from build123d import *

# Parameters (mm, degrees)
FILLET1_R = 1.27


with BuildPart() as part:
    # Sketch1 → Revolve-Thin1 (revolve)
    with BuildSketch(Plane(origin=(0, 0, 0), x_dir=(1, 0, 0), z_dir=(0, 1, 0)), mode=Mode.PRIVATE) as revolve_thin1_sk:
        Polygon((-77.419354839, 0), (-77.419354839, 3.5), (-67.870967742, 3.5), (-67.870967742, 4), (-57.608712258, 4), (-57.608712258, 6.35), (67.904423226, 6.35), (67.904423226, 4), (76.082332903, 4), (76.082332903, 3.5), (87.741935484, 3.5), (87.741935484, 0), (85.201935484, 0), (85.201935484, 0.96), (73.542332903, 0.96), (73.542332903, 1.46), (65.364423226, 1.46), (65.364423226, 3.81), (-55.068712258, 3.81), (-55.068712258, 1.46), (-65.330967742, 1.46), (-65.330967742, 0.96), (-74.879354839, 0.96), (-74.879354839, 0), align=None)
    revolve(revolve_thin1_sk.sketch.rotate(Axis((-77.419354839, 0, 0), (1, 0, 0)), 180), axis=Axis((-77.419354839, 0, 0), (1, 0, 0)))

    # Fillet1
    # the kernel refuses this fillet: 1.27 mm, written as the material it adds along each edge
    with BuildSketch(Plane(origin=(-67.870967742, 0, 0), x_dir=(0, 0, 1), z_dir=(0, 1, 0))) as fillet1_piece_1:
        with BuildLine():
            CenterArc((4.77, -1.009950494), FILLET1_R, 127.322390296, 52.677609704)
            Line((4, 0), (3.9846, 0.02019901))
            ThreePointArc((3.9846, 0.02019901), (3.75, 0.0254), (3.5, 0.0254))
            Line((3.5, 0.0254), (3.4746, 0))
            Line((3.4746, 0), (3.4746, -1.009950494))
            Line((3.4746, -1.009950494), (3.5, -1.009950494))
        make_face()
    revolve(axis=Axis((-67.870967742, 0, 0), (1, 0, 0)))
    with BuildSketch(Plane(origin=(-57.608712258, 0, 0), x_dir=(0, 0, 1), z_dir=(0, 1, 0))) as fillet1_piece_2:
        with BuildLine():
            CenterArc((4 + FILLET1_R, -FILLET1_R), FILLET1_R, 90, 90)
            Line((4 + FILLET1_R, 0), (4 + FILLET1_R, FILLET1_R * 0.02))
            Line((4 + FILLET1_R, FILLET1_R * 0.02), (4 - FILLET1_R * 0.02, FILLET1_R * 0.02))
            Line((4 - FILLET1_R * 0.02, FILLET1_R * 0.02), (4 - FILLET1_R * 0.02, -FILLET1_R))
            Line((4 - FILLET1_R * 0.02, -FILLET1_R), (4, -FILLET1_R))
        make_face()
    revolve(axis=Axis((-57.608712258, 0, 0), (1, 0, 0)))
    with BuildSketch(Plane(origin=(67.904423226, 0, 0), x_dir=(0, 0, 1), z_dir=(0, 1, 0))) as fillet1_piece_3:
        with BuildLine():
            CenterArc((4 + FILLET1_R, FILLET1_R), FILLET1_R, 180, 90)
            Line((4, FILLET1_R), (4 - FILLET1_R * 0.02, FILLET1_R))
            Line((4 - FILLET1_R * 0.02, FILLET1_R), (4 - FILLET1_R * 0.02, -FILLET1_R * 0.02))
            Line((4 - FILLET1_R * 0.02, -FILLET1_R * 0.02), (4 + FILLET1_R, -FILLET1_R * 0.02))
            Line((4 + FILLET1_R, -FILLET1_R * 0.02), (4 + FILLET1_R, 0))
        make_face()
    revolve(axis=Axis((67.904423226, 0, 0), (1, 0, 0)))
    with BuildSketch(Plane(origin=(76.082332903, 0, 0), x_dir=(0, 0, 1), z_dir=(0, 1, 0))) as fillet1_piece_4:
        with BuildLine():
            CenterArc((4.77, 1.009950494), FILLET1_R, 180, 52.677609704)
            Line((3.5, 1.009950494), (3.4746, 1.009950494))
            Line((3.4746, 1.009950494), (3.4746, 0))
            Line((3.4746, 0), (3.5, -0.0254))
            ThreePointArc((3.5, -0.0254), (3.75, -0.0254), (3.9846, -0.02019901))
            Line((3.9846, -0.02019901), (4, 0))
        make_face()
    revolve(axis=Axis((76.082332903, 0, 0), (1, 0, 0)))


solid = part.part
The listing builds one solid part. Answer for the finished solid, in the listing's coordinates (mm). A direction names the side the tool comes from. Give positions to 0.01 mm unless a question says otherwise; leave off trailing zeros. Order: outer loops, then holes, each group sorted by start corner. A loop starts at its lowest first (then second) coordinate and runs counter-clockwise, first axis right, second up. Notation, with made-up numbers: (-23.5, 16.5) - (13.5, 16.5) arc R17 ccw to (13.5, 33.5) - close; hole circle Ø2 at (4, -10). An arc over 180 degrees is marked (long way). Answer as CSV lines item,"result".
Q1. Which of the six approach directions +Z, -Z, +X, -X, +Y, -Y give full straight-line access (tool end or side, diameter ignored) to faces 1 (the face through (-73.09, 1.341, 3.233)), 2 (the face through (87.742, 0, 0)), 3 (the face through (67.904, -4, -4)), 4 (the face through (69.396, -0.987, -1.076))?
Answer key:
face 1,"-X"
face 2,"+Z, -Z, +X, +Y, -Y"
face 3,"+X"
face 4,"none"
Q2. Straight lines are drawn through the part: L1, parallel to Z at x = 8.5, y = -0.25; L2, parallel to X at y = 3, z = 0; L3, parallel to Y at x = 81.25, z = 0. For each, find the intervals that lie inside material, in ascending order.
Answer key:
L1,"z = -6.35 to -3.8, 3.8 to 6.35"
L2,"x = -77.42 to -55.07, 65.36 to 87.74"
L3,"y = -3.5 to -0.96, 0.96 to 3.5"
Q3. Each of these flat-tipped pins is pushed along its axis until it touches: pin 1 Ø1.5 at (x, z) = (-32.5, 3.5) entering from -Y; pin 2 Ø1 at (x, y) = (16.5, -4.5) entering from -Z; pin 3 Ø2 at (y, z) = (2.5, -3) entering from +X; pin 4 Ø6 at (x, y) = (55.5, 5) entering from -Z. Where does it stop, or does it pass through?
Answer key:
pin 1,"stops at y = -5.72"
pin 2,"stops at z = -4.93"
pin 3,"stops at x = 87.74"
pin 4,"stops at z = -6.03"
Q4. Determine the mould class of faces 5 (the face through (6.026, 5.634, 2.93)), 6 (the face through (-57.609, -4, 4)), 7 (the face through (-60.272, -0.987, -1.076)) for opening direction Y: pulls with the +Y half, pulls with the -Y half, needs draft (parallel to the pull), parting line crosses it, or undercut.
Answer key:
face 5,"parting line crosses it"
face 6,"needs draft"
face 7,"undercut"
Q5. A cutting plane is placed at A-A, the plane x = -3. Determine the outline of the cut face in (y, z), and give its area (3 significant figures).
Answer key:
outline,"circle Ø12.7 at (0, 0); hole circle Ø7.62 at (0, 0)"
area,"81.1 mm^2"
